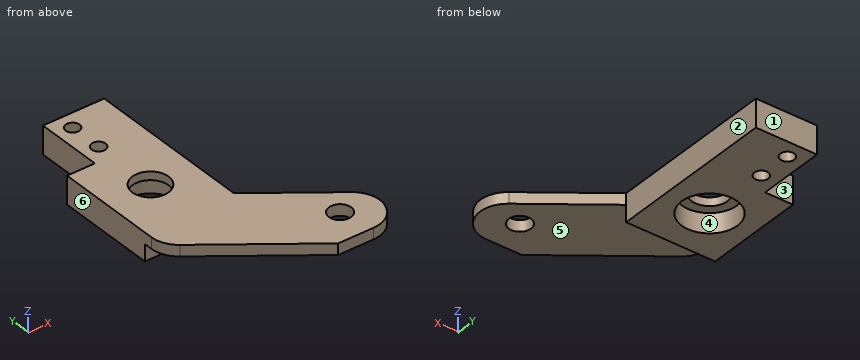
```python
from build123d import *

# Parameters (mm, degrees)
EXTRUDE1_DEPTH        = 5
SKETCH3_R             = 5
EXTRUDE3_DEPTH        = 3.5
SKETCH4_R             = 3.25
EXTRUDE4_DEPTH        = 1.5
SKETCH5_W             = 5
SKETCH5_H             = 12
EXTRUDE5_DEPTH        = 5
SKETCH6_R             = 1.25
EXTRUDE6_DEPTH        = 5
FILLET1_R             = 5
EXTRUDE7_START        = -3
EXTRUDE7_DEPTH        = 3
SKETCH8_R             = 2
EXTRUDE8_DEPTH        = 2
M3_TAPPED_HOLE1_D     = 2.5
M3_TAPPED_HOLE1_DEPTH = 8
M3_TAPPED_HOLE1_TIP   = 0.751075774


with BuildPart() as part:
    # Sketch1 → Extrude1 (new body)
    with BuildSketch(Plane.XY):
        Polygon((-8, -13), (12, -28), (33.333333333, -28), (8, -9), (8, 21), (-8, 21), align=None)
    extrude(amount=EXTRUDE1_DEPTH)

    # Sketch3 → Extrude3 (cut)
    with BuildSketch(Plane(origin=(0, 0, 0), x_dir=(-1, 0, 0), z_dir=(0, 0, -1))):
        Circle(SKETCH3_R)
    extrude(amount=-EXTRUDE3_DEPTH, mode=Mode.SUBTRACT)

    # Sketch4 → Extrude4 (cut)
    with BuildSketch(Plane(origin=(0, 0, 3.5), x_dir=(-1, 0, 0), z_dir=(0, 0, -1))):
        Circle(SKETCH4_R)
    extrude(amount=-EXTRUDE4_DEPTH, mode=Mode.SUBTRACT)

    # Sketch5 → Extrude5 (cut)
    with BuildSketch(Plane.XY.offset(5)):
        with Locations((-5.5, 15)):
            Rectangle(SKETCH5_W, SKETCH5_H)
    extrude(amount=-EXTRUDE5_DEPTH, mode=Mode.SUBTRACT)

    # Sketch6 → Extrude6 (cut)
    with BuildSketch(Plane(origin=(0, 0, 0), x_dir=(-1, 0, 0), z_dir=(0, 0, -1))):
        with Locations((0, 18)):
            Circle(SKETCH6_R)
        with Locations((0, 12)):
            Circle(SKETCH6_R)
    extrude(amount=-EXTRUDE6_DEPTH, mode=Mode.SUBTRACT)

    # Fillet1
    fillet1_edges = [part.edges().sort_by_distance(p)[0] for p in [
        (33.333333333, -28, 2.5),
        (-8, -13, 2.5),
    ]]
    fillet(fillet1_edges, radius=FILLET1_R)

    # Sketch7 → Extrude7 (cut)
    with BuildSketch(Plane(origin=(0, 0, 0), x_dir=(-1, 0, 0), z_dir=(0, 0, -1)).offset(EXTRUDE7_START)):
        with BuildLine():
            Line((-8, -9), (8, -9))
            Line((8, -9), (8, -10.5))
            ThreePointArc((8, -10.5), (7.472135955, -12.736067977), (6, -14.5))
            Line((6, -14.5), (-12, -28))
            Line((-12, -28), (-18.333333333, -28))
            ThreePointArc((-18.333333333, -28), (-23.076749824, -24.58113883), (-21.333333333, -19))
            Line((-21.333333333, -19), (-8, -9))
        make_face()
    extrude(amount=EXTRUDE7_DEPTH, mode=Mode.SUBTRACT)

    # Sketch8 → Extrude8 (cut)
    with BuildSketch(Plane(origin=(0, 0, 3), x_dir=(-1, 0, 0), z_dir=(0, 0, -1))):
        with Locations((-17, -22)):
            Circle(SKETCH8_R)
    extrude(amount=-EXTRUDE8_DEPTH, mode=Mode.SUBTRACT)

    # M3 Tapped Hole1
    with Locations(Plane(origin=(0, 18, 0), x_dir=(-1, 0, 0), z_dir=(0, 0, -1))):
        with Locations((0, 0), (0, -6)):
            Hole(M3_TAPPED_HOLE1_D / 2, depth=M3_TAPPED_HOLE1_DEPTH)
            with Locations((0, 0, -(M3_TAPPED_HOLE1_DEPTH + M3_TAPPED_HOLE1_TIP / 2))):  # 118° drill point
                Cone(0, M3_TAPPED_HOLE1_D / 2, M3_TAPPED_HOLE1_TIP, mode=Mode.SUBTRACT)


solid = part.part
```
Check sheet for the modelled part. Datum: model origin and axes. Units: mm. Face numbers are marked on the shaded views. A direction names the side the tool comes from. Give positions to 0.01 mm unless a question says otherwise; leave off trailing zeros. Order: outer loops, then holes, each group sorted by start corner. A loop starts at its lowest first (then second) coordinate and runs counter-clockwise, first axis right, second up. Notation, with made-up numbers: M 24.25,5 L 35.25,5 A12 ccw 35.25,21 Z; hole C -27,84 d7. An arc over 180 degrees is marked long. Answer in a Markdown table with one row per item.
1) Cross-section at A-A, the plane x = 0. Enter the section's corners in (y, z), plus the area to 3 significant figures.
Filled sheet:
| item | result |
|---|---|
| outline | M -19,3 L -9,3 L -9,0 L -5,0 L -5,3.5 L -3.25,3.5 L -3.25,5 L -19,5 Z; M 3.25,3.5 L 5,3.5 L 5,0 L 10.75,0 L 10.75,5 L 3.25,5 Z; M 13.25,0 L 16.75,0 L 16.75,5 L 13.25,5 Z; M 19.25,0 L 21,0 L 21,5 L 19.25,5 Z |
| area | 100 mm2 |
2) Cross-section at B-B, the plane y = 0. Enter the section's corners in (x, z).
Filled sheet:
| item | result |
|---|---|
| outline | M -8,0 L -5,0 L -5,3.5 L -3.25,3.5 L -3.25,5 L -8,5 Z; M 3.25,3.5 L 5,3.5 L 5,0 L 8,0 L 8,5 L 3.25,5 Z |
3) Access from +Z, -Z, +X, -X, +Y, -Y to the whole of each face (thin tool, end or side, straight path). Record for the marked faces 1, 2 and 3.
Filled sheet:
| item | result |
|---|---|
| face 1 | +Z, -Z, +X, -X, +Y |
| face 2 | +Z, -Z, +X, +Y |
| face 3 | +Z, -Z, -X, +Y |
4) Cross-section at C-C, the plane x = 17. Enter the section's corners in (y, z).
Filled sheet:
| item | result |
|---|---|
| outline | M -28,3 L -24,3 L -24,5 L -28,5 Z; M -20,3 L -15.75,3 L -15.75,5 L -20,5 Z |
5) Thickness scan on L1, parallel to Y at x = 0, z = 3.45; L2, parallel to Y at x = 0, z = 4.1; L3, parallel to Y at x = -4, z = 2.4. Record the ranges inside material, lowest first. Write a range as [from, to].
Filled sheet:
| item | result |
|---|---|
| L1 | y = [-19, -5], [5, 10.75], [13.25, 16.75], [19.25, 21] |
| L2 | y = [-19, -3.25], [3.25, 10.75], [13.25, 16.75], [19.25, 21] |
| L3 | y = [-9, -3], [3, 9] |
6) Release check for a two-part mould opening along X. For the marked faces 4, 5 and 6 record: +X half, -X half, draft (parallel to the pull), parting line (faces both ways), or undercut.
Filled sheet:
| item | result |
|---|---|
| face 4 | undercut |
| face 5 | draft |
| face 6 | -X half |
7) Gauge pin test, flat ends, axial feed: P1, Ø2.5, axis at y = 16, z = 2.5, coming from the -X side; P2, Ø2.5, axis at y = 4.5, z = 3, coming from the +X side; P3, Ø2, axis at x = 0, y = 18, coming from the -Z side; P4, Ø1.5, axis at x = 3, z = 0.5, coming from the -Y side. Record the tip position at first contact, or that the pin passes through.
Filled sheet:
| item | result |
|---|---|
| P1 | stops at x = -3 |
| P2 | stops at x = 8 |
| P3 | passes through |
| P4 | stops at y = -9 |
8) Cross-section at D-D, the plane z = 0.7. Enter the section's corners in (x, y), plus the area to 3 significant figures.
Filled sheet:
| item | result |
|---|---|
| outline | M -8,-9 L 8,-9 L 8,21 L -3,21 L -3,9 L -8,9 Z; hole C 0,0 d10; hole C 0,12 d2.5; hole C 0,18 d2.5 |
| area | 332 mm2 |
